from build123d import *

# Parameters (mm, degrees)
CHAMFER1_SIZE  = 3
CHAMFER2_SIZE  = 0.2
CHAMFER2_SIZE2 = 0.549495484
CHAMFER3_SIZE  = 0.4
CHAMFER3_SIZE2 = 0.476701437


with BuildPart() as part:
    # Sketch1 → Revolve1 (revolve)
    with BuildSketch(Plane.XY):
        Polygon((0, 0), (3.75, 0), (3.75, 6.35), (12, 6.35), (12, 18), (6.7, 18), (6.7, 10), (0, 10), align=None)
    revolve(axis=Axis((0, 10, 0), (0, -1, 0)))

    # Chamfer1
    chamfer1_edges = [part.edges().sort_by_distance(p)[0] for p in [
        (-6.7, 10, 0),
    ]]
    chamfer(chamfer1_edges, length=CHAMFER1_SIZE)

    # Chamfer2
    chamfer2_edges = [part.edges().sort_by_distance(p)[0] for p in [
        (-3.75, 0, 0),
    ]]
    chamfer2_side = [part.faces().sort_by_distance(p)[0] for p in [
        (0, 0, 0),
    ]]
    chamfer(chamfer2_edges, length=CHAMFER2_SIZE, length2=CHAMFER2_SIZE2, reference=chamfer2_side[0])

    # Chamfer3
    chamfer3_edges = [part.edges().sort_by_distance(p)[0] for p in [
        (-6.7, 18, 0),
    ]]
    chamfer3_side = [part.faces().sort_by_distance(p)[0] for p in [
        (-11.660588745, 18, 0),
    ]]
    chamfer(chamfer3_edges, length=CHAMFER3_SIZE, length2=CHAMFER3_SIZE2, reference=chamfer3_side[0])


solid = part.part
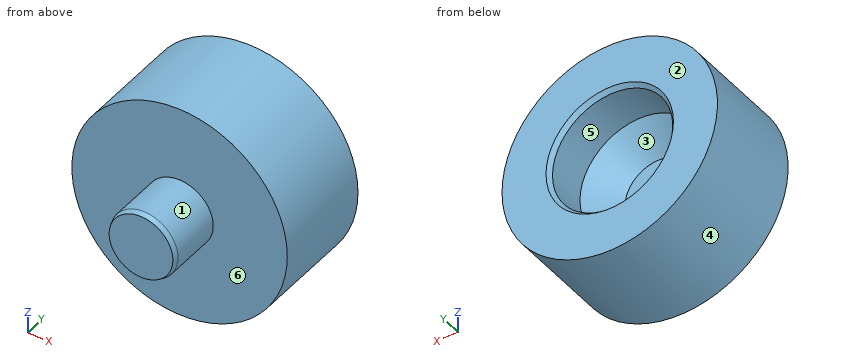
Source: CAD feature listing. Evaluate the final solid. Frame: model axes, mm. Face numbers are marked on the shaded views. A direction names the side the tool comes from. Coordinates: 2 decimals unless noted, no trailing zeros. Loops run counter-clockwise (first coordinate to the right, second up) from the corner with the lowest first, then second, coordinate; pieces in that order, holes last. Notation, with made-up numbers: (42, 85.25) -> (46, 85.25) arc R10 cw to (46, 98.25) -> close; hole circle Ø5 at (29, -36). An arc over 180 degrees is marked (long way). Answer in a Markdown table with one row per item. Add a question column.
Q1. Ray query, line 1 along Z through (x, y) = (0, 15.4); line 2 along Y through (x, z) = (-4.75, 6.75); line 3 along X through (y, z) = (14.25, 5.25). Return the intervals inside material, ascending.
Q2. Section A-A on z = 0. Return the cut outline in (x, y).
Q3. Contact query for flat-ended pins moving along their axis: pin 1 Ø6 at (y, z) = (2, -1.5) entering from +X; pin 2 Ø8 at (x, z) = (8.5, 4.5) entering from -Y; pin 3 Ø2 at (x, z) = (-0.5, -0.5) entering from +Y. Output: stop coordinate, or through.
Q4. Section D-D on y = 8.5. Return the cut outline in (x, z).
Q5. Section B-B on x = 0. Return the cut outline in (y, z), and give its area (3 significant figures).
Q6. Reachability of the marked faces 4, 5 and 6 from +Z, -Z, +X, -X, +Y, -Y: full face, straight path, thin tool, end or side. Return the list, or none.
Q7. Pull-direction query (X, two-part tool) for the marked faces 1, 2 and 3; classes: pulls with the +X half, pulls with the -X half, needs draft (parallel to the pull), parting line crosses it, or undercut.
Q8. Section C-C on y = 14.75. Return the cut outline in (x, z).
Computed values:
| question | item | result |
|---|---|---|
| 1 | line 1 | z = -12 to -6.7, 6.7 to 12 |
| 1 | line 2 | y = 6.35 to 18 |
| 1 | line 3 | x = -10.79 to -4.16, 4.16 to 10.79 |
| 2 | outline | (-12, 6.35) -> (-3.75, 6.35) -> (-3.75, 0.55) -> (-3.55, 0) -> (3.55, 0) -> (3.75, 0.55) -> (3.75, 6.35) -> (12, 6.35) -> (12, 18) -> (7.1, 18) -> (6.7, 17.52) -> (6.7, 13) -> (3.7, 10) -> (-3.7, 10) -> (-6.7, 13) -> (-6.7, 17.52) -> (-7.1, 18) -> (-12, 18) -> close |
| 3 | pin 1 | stops at x = 3.75 |
| 3 | pin 2 | stops at y = 6.35 |
| 3 | pin 3 | stops at y = 10 |
| 4 | outline | circle Ø24 at (0, 0) |
| 5 | outline | (0, -3.55) -> (0.55, -3.75) -> (6.35, -3.75) -> (6.35, -12) -> (18, -12) -> (18, -7.1) -> (17.52, -6.7) -> (13, -6.7) -> (10, -3.7) -> (10, 3.7) -> (13, 6.7) -> (17.52, 6.7) -> (18, 7.1) -> (18, 12) -> (6.35, 12) -> (6.35, 3.75) -> (0.55, 3.75) -> (0, 3.55) -> close |
| 5 | area | 229 mm^2 |
| 6 | face 4 | +Y, -Y |
| 6 | face 5 | +Y |
| 6 | face 6 | -Y |
| 7 | face 1 | parting line crosses it |
| 7 | face 2 | needs draft |
| 7 | face 3 | undercut |
| 8 | outline | circle Ø24 at (0, 0); hole circle Ø13.4 at (0, 0) |
